Can you work these out from the model? Positions are in its coordinate system, mm. A direction names the side the tool comes from. Give positions to 0.01 mm unless a question says otherwise; leave off trailing zeros. Loops run counter-clockwise (first coordinate to the right, second up) from the corner with the lowest first, then second, coordinate; pieces in that order, holes last. Notation, with made-up numbers: M 60,-0.5 L 117,-0.5 A14 cw 117,7.5 Z; hole C 30,13 d9. An arc over 180 degrees is marked long. Put each result on its own line as item: value. Start each with the question number.
1) For P1, Ø0.8, axis at x = 166, y = 8.5, coming from the -Z side; P2, Ø0.8, axis at x = 160, y = 8, coming from the +Z side; P3, Ø4, axis at y = 0, z = 0, coming from the -X side, each with a flat end and sliding along its axis, tell me the tip position at first contact or that it passes through.
2) For faces 1 (the cylindrical face through (145, 9, 0)), 2 (the cylindrical face through (60, 9, 0)), 3 (the cylindrical face through (25.35, 9.76, 2.17)), which set-ups out of +Z, -Z, +X, -X, +Y, -Y let a thin tool reach every point of the face, with its end or its side?
3) Imagine slicing it at B-B (x = 110). Write out the boundary of the cut face in (y, z), then the cut area to 3 significant figures.
4) Please list where these lines run through material, in increasing order: line 1 along Z through (x, y) = (168, 0); line 2 along Z through (x, y) = (110.5, 0.5). Write a range as from..to.
5) Imagine slicing it at A-A (z = -5). Write out the boundary of the cut face in (x, y), then the cut area to 3 significant figures.
6) If we mould it in two halves opening along X, with no side actions, what happens to faces 4 (the cylindrical face through (85, 9, 0)), 5 (the flat face through (0, 2, 2)), 6 (the cylindrical face through (5.08, 2.44, -0.54)), 7 (the flat face through (73, 7, 0))? For each: +X half, -X half, draft (parallel to the pull), parting line (faces both ways), or undercut.
7) Imagine slicing it at C-C (y = -5.75). Write out the boundary of the cut face in (x, z), then the cut area to 3 significant figures.
from build123d import *

# Parameters (mm, degrees)
F_5_0MM_DOWEL_HOLE1_D           = 5
F_5_0MM_DOWEL_HOLE1_DEPTH       = 10
F_5_0MM_DOWEL_HOLE1_CSINK_D     = 5.05
F_5_0MM_DOWEL_HOLE1_CSINK_ANGLE = 90
F_5_0MM_DOWEL_HOLE1_TIP         = 1.502151548
CUT_EXTRUDE1_DEPTH              = 3


with BuildPart() as part:
    # Sketch1 → Revolve1 (revolve)
    with BuildSketch(Plane(origin=(0, 0, 0), x_dir=(1, 0, 0), z_dir=(0, 1, 0))):
        Polygon((0, 0), (0, 10), (50, 10), (50, 12.5), (60, 12.5), (60, 10), (175, 10), (175, 0), align=None)
    revolve(axis=Axis((175, 0, 0), (-1, 0, 0)))

    # Ø5.0mm Dowel Hole1
    with Locations(Plane(origin=(0, 0, 0), x_dir=(0, 0, -1), z_dir=(-1, 0, 0))):
        with Locations((0, 0)):
            CounterSinkHole(F_5_0MM_DOWEL_HOLE1_D / 2, F_5_0MM_DOWEL_HOLE1_CSINK_D / 2, depth=F_5_0MM_DOWEL_HOLE1_DEPTH, counter_sink_angle=F_5_0MM_DOWEL_HOLE1_CSINK_ANGLE)
            with Locations((0, 0, -(F_5_0MM_DOWEL_HOLE1_DEPTH + F_5_0MM_DOWEL_HOLE1_TIP / 2))):  # 118° drill point
                Cone(0, F_5_0MM_DOWEL_HOLE1_D / 2, F_5_0MM_DOWEL_HOLE1_TIP, mode=Mode.SUBTRACT)

    # Sketch9 → Ø5.0mm Dowel Hole2 (revolve, cut)
    with BuildSketch(Plane(origin=(175, 0, 0), x_dir=(0, 0, -1), z_dir=(0, 1, 0))):
        Polygon((0, 0), (0, 11.502151548), (2.5, 10), (2.5, 0.025), (2.525, 0), align=None)
    revolve(axis=Axis((181.35, 0, 0), (-1, 0, 0)), mode=Mode.SUBTRACT)

    # Sketch10 → Cut-Extrude1 (cut)
    with BuildSketch(Plane(origin=(0, 10, 0), x_dir=(1, 0, 0), z_dir=(0, 1, 0))):
        with BuildLine():
            Line((63, 3), (82, 3))
            ThreePointArc((82, 3), (85, 0), (82, -3))
            Line((82, -3), (63, -3))
            ThreePointArc((63, -3), (60, 0), (63, 3))
        make_face()
        with BuildLine():
            Line((175, -3), (148, -3))
            ThreePointArc((148, -3), (145, 0), (148, 3))
            Line((148, 3), (175, 3))
            ThreePointArc((175, 3), (178, 0), (175, -3))
        make_face()
    extrude(amount=-CUT_EXTRUDE1_DEPTH, mode=Mode.SUBTRACT)


solid = part.part
Recorded:
1. P1: z = -5.86
1. P2: z = 6.5
1. P3: x = 10.3
2. face 1: +X, +Y
2. face 2: +Y
2. face 3: -X
3. outline: C 0,0 d20
3. area: 314 mm²
4. line 1: -10..-2.5, 2.5..10
4. line 2: -9.99..9.99
5. outline: M 0,-8.66 L 50,-8.66 L 50,-11.46 L 60,-11.46 L 60,-8.66 L 175,-8.66 L 175,8.66 L 60,8.66 L 60,11.46 L 50,11.46 L 50,8.66 L 0,8.66 Z
5. area: 3,090 mm²
6. face 4: undercut
6. face 5: -X half
6. face 6: draft
6. face 7: undercut
7. outline: M 0,-8.18 L 50,-8.18 L 50,-11.1 L 60,-11.1 L 60,-8.18 L 175,-8.18 L 175,8.18 L 60,8.18 L 60,11.1 L 50,11.1 L 50,8.18 L 0,8.18 Z
7. area: 2,920 mm²
